The listing builds one solid part. Answer for the finished solid, in the listing's coordinates (mm). A direction names the side the tool comes from. Give positions to 0.01 mm unless a question says otherwise; leave off trailing zeros. Write each loop counter-clockwise with the first axis right and the second up, starting at its lowest first coordinate (ties: lowest second). Pieces come first, ordered by that corner, then holes. Notation, with made-up numbers: (16, 11.25) - (29, 11.25) arc R30 cw to (29, 50.25) - close; hole circle Ø4 at (48.25, 34.25). An arc over 180 degrees is marked (long way). Return JSON: item names as keys, results as strings.
from build123d import *

# Parameters (mm, degrees)
F4_R      = 3.6618559104
F5_DEPTH  = 16.256
F6_R      = 1.7816904606
F7_DEPTH  = 27.178
F8_R      = 1.1877343137
F9_DEPTH  = 72.136
F10_R     = 1.6542577125
F11_DEPTH = 132.588


# Not quite as in the source:
# - the program builds the solid bodies; features that only make, move or delete a surface that nothing else refers to are left out


with BuildPart() as f1:
    # F0 (on Front) → F1 (revolve)
    with BuildSketch(Plane.XZ):
        with BuildLine():
            Line((0, 22.9268427938), (0, 0))
            ThreePointArc((0, 0), (9.3672569036, 11.4634213969), (0, 22.9268427938))
        make_face()
    revolve(axis=Axis((0, 0, 11.4634213969), (0, 0, 1)))

    # F4 (on Front) → F5 (join)
    with BuildSketch(Plane.XZ):
        with Locations((4.9128951505, 10.7615785673)):
            Circle(F4_R)
    extrude(amount=-F5_DEPTH)

    # F6 (on Top) → F7 (join)
    with BuildSketch(Plane.XY):
        Circle(F6_R)
    extrude(amount=F7_DEPTH)

    # F8 (on Right) → F9 (cut)
    with BuildSketch(Plane.YZ):
        with Locations((0, 24.8752553016)):
            Circle(F8_R)
    extrude(amount=-F9_DEPTH, mode=Mode.SUBTRACT)

    # F10 (on Right) → F11 (cut)
    with BuildSketch(Plane.YZ):
        with Locations((0, 24.7984230518)):
            Circle(F10_R)
    extrude(amount=F11_DEPTH, mode=Mode.SUBTRACT)


solid = f1.part
Item 1: For faces 1 (the face through (8.296, 11.281, 9.359)), 2 (the face through (1.699, 0.535, 0.252)), 3 (the face through (0.68, 0.889, 26.193)), 4 (the face through (-0.39, -1.74, 24.76)), 5 (the face through (5, 16.256, 11)), determine the directions among +Z, -Z, +X, -X, +Y, -Y from which every point of the face is accessible in a straight line to the end or side of a thin tool.
Answer below:
{"face 1": "+Y", "face 2": "-Z", "face 3": "+X", "face 4": "+Z", "face 5": "+Z, -Z, +X, -X, +Y"}
Item 2: Consider L1, parallel to Z at x = 1.1, y = 0; L2, parallel to X at y = -1.75, z = 21.5; L3, parallel to X at y = 9, z = 8. Determine where each line is inside the solid, lowest interval first.
Answer below:
{"L1": "z = 0 to 23.14, 26.45 to 27.18", "L2": "x = -3.24 to 3.24", "L3": "x = 2.51 to 7.32"}
Item 3: A cutting plane is placed at A-A on y = 14.25. Determine the outline of the cut face in (x, z), then the cut area to 3 significant figures.
Answer below:
{"outline": "circle Ø7.32 at (4.91, 10.76)", "area": "42.1 mm²"}
Item 4: Flat-ended cylindrical pins translate along their axes: P1, Ø12, axis at y = 7.5, z = 8.5, coming from the -X side; P2, Ø1, axis at x = 6.5, y = 4.5, coming from the -Z side; P3, Ø2.5, axis at y = -0.5, z = 24, coming from the +X side; P4, Ø2, axis at y = 0, z = 24.88, coming from the -X side. Find the tip coordinate at first contact, or state that the pin passes through.
Answer below:
{"P1": "stops at x = -9.14", "P2": "stops at z = 4.98", "P3": "stops at x = 1.78", "P4": "passes through"}
